Answer from the drawing. Dimensions are ordinates in mm from the lowest x, y and z of the part. Coordinates: 2 decimals unless noted, no trailing zeros. Loops run counter-clockwise (first coordinate to the right, second up) from the corner with the lowest first, then second, coordinate; pieces in that order, holes last. Notation, with made-up numbers: M 14.5,-21.75 L 24.5,-21.75 A29 ccw 24.5,16.25 Z; hole C 60.5,88 d4. An arc over 180 degrees is marked long. Put each result on its own line as item: value.
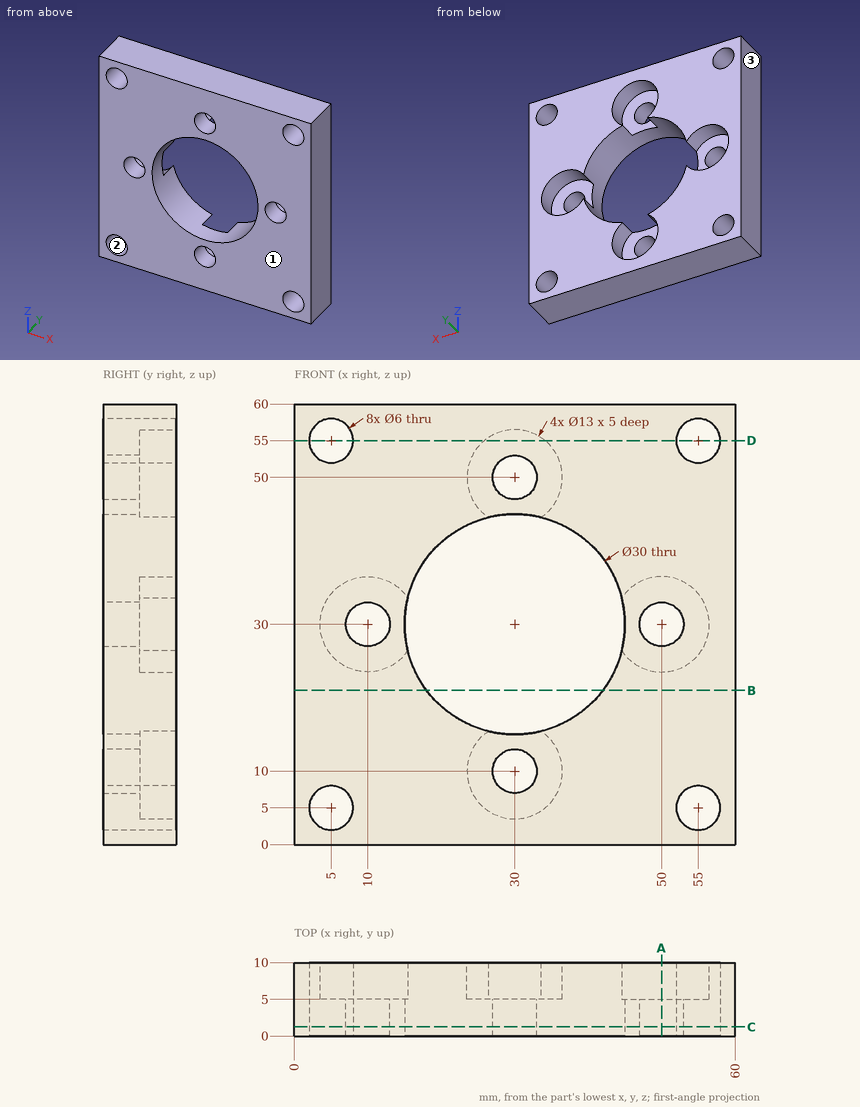
1) Find section D-D, the plane z = 55. Write down the section's boundary in (x, y).
Answer list:
outline: M 0,0 L 2,0 L 2,10 L 0,10 Z; M 8,0 L 52,0 L 52,10 L 34.15,10 L 34.15,5 L 25.85,5 L 25.85,10 L 8,10 Z; M 58,0 L 60,0 L 60,10 L 58,10 Z
2) Determine the mould class of the marked faces 1, 2 and 3 for opening direction X: released by +X, released by -X, zero draft, split by the parting line, or undercut.
Answer list:
face 1: zero draft
face 2: undercut
face 3: released by -X
3) Given pin 1 Ø5.5 at (x, z) = (5, 5) entering from -Y; pin 2 Ø3.5 at (x, z) = (53.5, 30.5) entering from +Y, each flat-ended and moving along its own axis, determine where each tip first touches the part or whether it passes through.
Answer list:
pin 1: passes through
pin 2: stops at y = 5
4) Find section A-A, the plane x = 50. Write down the section's boundary in (y, z).
Answer list:
outline: M 0,0 L 10,0 L 10,23.5 L 5,23.5 L 5,27 L 0,27 Z; M 0,33 L 5,33 L 5,36.5 L 10,36.5 L 10,60 L 0,60 Z
5) Straight lines are drawn through the part: line 1 (X direction, y = 4, z = 5); line 2 (Z direction, x = 30, y = 8.7); line 3 (X direction, y = 7.25, z = 55). For each, find the intervals that lie inside material, in ascending order. Write a range as [from, to].
Answer list:
line 1: x = [0, 2], [8, 52], [58, 60]
line 2: z = [0, 3.5], [56.5, 60]
line 3: x = [0, 2], [8, 25.85], [34.15, 52], [58, 60]
6) Find section B-B, the plane z = 21. Write down the section's boundary in (x, y).
Answer list:
outline: M 0,0 L 18,0 L 18,10 L 0,10 Z; M 42,0 L 60,0 L 60,10 L 42,10 Z
7) Find section C-C, the plane y = 1.25. Count the separate pieces of the cut face and the enclosed holes in it, plus the area to 3 significant figures.
Answer list:
separate pieces: 1
enclosed holes: 9
area: 2,670 mm^2
